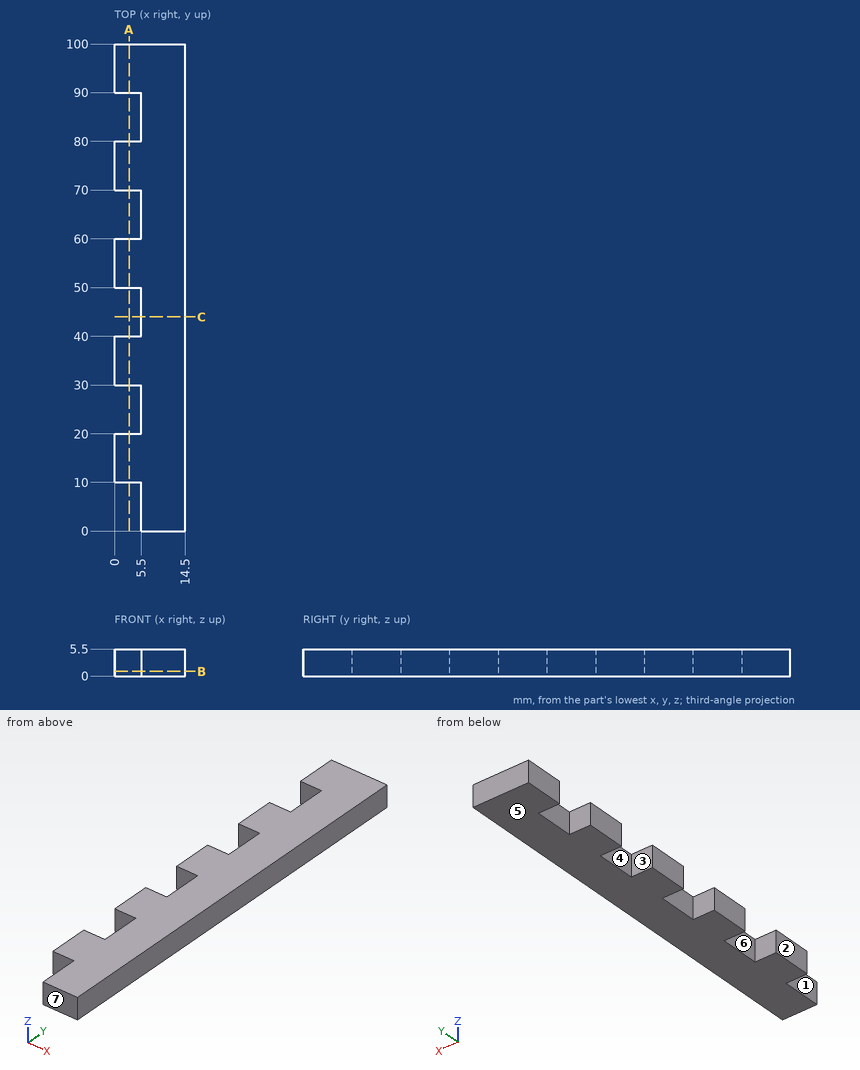
Print and shaded views of the part. All mm, measured from the part's lowest x, y and z. A direction names the side the tool comes from. Give positions to 0.01 mm unless a question says otherwise; leave off trailing zeros. Write each loop counter-clockwise with the first axis right and the second up, starting at its lowest first coordinate (ties: lowest second). Pieces come first, ordered by that corner, then holes. Notation, with made-up numbers: (57, 83.25) -> (95, 83.25) arc R17 ccw to (95, 105.25) -> close; hole circle Ø11 at (64, -21). An arc over 180 degrees is marked (long way). Use CSV: the item, a comma, the result in double quotes. Start each with the question number.
1) Cut at A-A on x = 3. List the corners of the cut face in (y, z), plus the area to 3 significant figures.
2) Pin check, flat tips, straight feed: P1, Ø3, axis at y = 63, z = 2, coming from the -X side; P2, Ø1.6, axis at x = 3.5, z = 4, coming from the -Y side. Stop position of each tip, or through.
3) Cut at C-C on y = 44. List the corners of the cut face in (x, z), plus the area to 3 significant figures.
4) Cut at B-B on z = 0.95. List the corners of the cut face in (x, y).
5) Drill centre lines: L1, parallel to Y at x = 1.5, z = 2.7; L2, parallel to X at y = 41, z = 4.55. Where is each one in solid material? Low to high.
6) Tool access for the marked faces 1, 2 and 3: list every direction of +Z, -Z, +X, -X, +Y, -Y with a clear straight run to the whole face (end or side of a thin tool).
7) Two-plate mould, pull along Y, no slides. Class the marked faces 4, 5, 6 and 7: released by +Y, released by -Y, zero draft, split by the parting line, or undercut.
Final values:
1,outline,"(10, 0) -> (20, 0) -> (20, 5.5) -> (10, 5.5) -> close; (30, 0) -> (40, 0) -> (40, 5.5) -> (30, 5.5) -> close; (50, 0) -> (60, 0) -> (60, 5.5) -> (50, 5.5) -> close; (70, 0) -> (80, 0) -> (80, 5.5) -> (70, 5.5) -> close; (90, 0) -> (100, 0) -> (100, 5.5) -> (90, 5.5) -> close"
1,area,"275 mm2"
2,P1,"stops at x = 5.5"
2,P2,"stops at y = 10"
3,outline,"(5.5, 0) -> (14.5, 0) -> (14.5, 5.5) -> (5.5, 5.5) -> close"
3,area,"49.5 mm2"
4,outline,"(0, 10) -> (5.5, 10) -> (5.5, 0) -> (14.5, 0) -> (14.5, 100) -> (0, 100) -> (0, 90) -> (5.5, 90) -> (5.5, 80) -> (0, 80) -> (0, 70) -> (5.5, 70) -> (5.5, 60) -> (0, 60) -> (0, 50) -> (5.5, 50) -> (5.5, 40) -> (0, 40) -> (0, 30) -> (5.5, 30) -> (5.5, 20) -> (0, 20) -> close"
5,L1,"y = 10 to 20, 30 to 40, 50 to 60, 70 to 80, 90 to 100"
5,L2,"x = 5.5 to 14.5"
6,face 1,"+Z, -Z, -X, -Y"
6,face 2,"+Z, -Z, -X, +Y, -Y"
6,face 3,"+Z, -Z, -X"
7,face 4,"undercut"
7,face 5,"zero draft"
7,face 6,"undercut"
7,face 7,"released by -Y"
